Geometry check sheet. Reference: the model listing, model coordinates, mm. A direction names the side the tool comes from. Round coordinates to 2 decimals unless told otherwise and drop trailing zeros. Order: outer loops, then holes, each group sorted by start corner. A loop starts at its lowest first (then second) coordinate and runs counter-clockwise, first axis right, second up. Notation, with made-up numbers: (23, 66.5) -> (31, 66.5) arc R16 ccw to (31, 83.5) -> close; hole circle Ø4 at (85.5, -6). An arc over 180 degrees is marked (long way). Answer as a JSON object with one key per item and string values. Group by question number.
from build123d import *

# Parameters (mm, degrees)
SKETCH1_W                  = 127.078191072
SKETCH1_H                  = 113.282646321
BOSS_EXTRUDE1_DEPTH        = 39.624
SHELL_1_T                  = -2.54
OFFICIAL_RIB_BLOCK20_DEPTH = 2.54


# Read off the part's stored shape, not the designer's step: official_rib_block20
with BuildPart() as part:
    # Sketch1 → Boss-Extrude1 (new body)
    with BuildSketch(Plane(origin=(0, 0, 0), x_dir=(1, 0, 0), z_dir=(0, 1, 0))):
        with Locations((1.06119575, 7.295720781)):
            Rectangle(SKETCH1_W, SKETCH1_H)
    extrude(amount=BOSS_EXTRUDE1_DEPTH)

    # 抽壳1
    shell_1_openings = [part.faces().sort_by_distance(p)[0] for p in [
        (1.06119575, 39.624, -7.295720782),
    ]]
    offset(amount=SHELL_1_T, openings=shell_1_openings, kind=Kind.INTERSECTION)

    # official_rib_block20 outline → official_rib_block20 (add)
    with BuildSketch(Plane(origin=(0.729572078, 0, -0.729572078), x_dir=(0.7071067811865477, 0, 0.7071067811865475), z_dir=(-0.7071067811865475, 0, 0.7071067811865477))):
        Polygon((67.224888407, 33.535890054), (7.726, 25.357), (-34.23, 35.134), (-85.796761505, 21.08206499), (-86, 21.02668253), (-86, 2), (68, 2), (68, 33.642439145), align=None)
    extrude(amount=OFFICIAL_RIB_BLOCK20_DEPTH)


solid = part.part
Item 1: Sectioned sample at C-C, the plane x = 20. Enter the section's corners in (y, z), then the cut area to 3 significant figures.
Item 2: Set-up check for faces 5 (the flat face through (-9.319, 30.177, -9.007)), 6 (the flat face through (0, 20, 49.346)): record each of +Z, -Z, +X, -X, +Y, -Y from which the full face is reachable in a straight line by a thin tool's end or side.
Item 3: Sectioned sample at A-A, the plane y = 7. Enter the section's corners in (x, z).
Item 4: Thickness scan on L1, parallel to Z at x = 33, y = 14.5; L2, parallel to Z at x = 21.5, y = 8; L3, parallel to X at y = 9.5, z = 20. Record the ranges inside material, lowest first.
Item 5: Sectioned sample at D-D, the plane z = 22. Enter the section's corners in (x, y), then the cut area to 3 significant figures.
Item 6: Depth check by flat-ended pin: pin 1 Ø2 at (x, z) = (48.5, 26) entering from +Y. Enter the tip coordinate at first touch or a pass-through.
Item 7: Sectioned sample at B-B, the plane y = 27. Enter the section's corners in (x, z), then the cut area to 3 significant figures.
Item 8: Mould release check, pull along X, two halves, no side actions. Record for faces 1 (the flat face through (-59.938, 21, -7)), 2 (the flat face through (0, 20, -63.937)), 3 (the flat face through (-32, 2.54, 17)), 4 (the flat face through (64.6, 20, -7)): pulls with the +X half, pulls with the -X half, needs draft (parallel to the pull), parting line crosses it, or undercut.
Result:
{
 "1": {"outline": "(0, -63.94) -> (39.62, -63.94) -> (39.62, -61.4) -> (2.54, -61.4) -> (2.54, 18.54) -> (28.04, 18.54) -> (28.39, 22.13) -> (2.54, 22.13) -> (2.54, 46.81) -> (39.62, 46.81) -> (39.62, 49.35) -> (0, 49.35) -> close", "area": "568 mm2"},
 "2": {"face 5": "+Y", "face 6": "+Z, +X, -X, +Y, -Y"},
 "3": {"outline": "(-62.48, -63.94) -> (64.6, -63.94) -> (64.6, 49.35) -> (-62.48, 49.35) -> close; hole (-59.94, -61.4) -> (62.06, -61.4) -> (62.06, 46.81) -> (48.26, 46.81) -> close; hole (-59.94, -57.8) -> (44.67, 46.81) -> (-59.94, 46.81) -> close"},
 "4": {"L1": "z = -63.94 to -61.4, 31.54 to 35.13, 46.81 to 49.35", "L2": "z = -63.94 to -61.4, 20.04 to 23.63, 46.81 to 49.35", "L3": "x = -62.48 to -59.94, 17.87 to 21.46, 62.06 to 64.6"},
 "5": {"outline": "(-62.48, 0) -> (64.6, 0) -> (64.6, 39.62) -> (62.06, 39.62) -> (62.06, 2.54) -> (23.46, 2.54) -> (23.46, 28.71) -> (19.87, 28.36) -> (19.87, 2.54) -> (-59.94, 2.54) -> (-59.94, 39.62) -> (-62.48, 39.62) -> close", "area": "605 mm2"},
 "6": {"pin 1": "stops at y = 2.54"},
 "7": {"outline": "(-62.48, -63.94) -> (64.6, -63.94) -> (64.6, 49.35) -> (-62.48, 49.35) -> close; (-46.38, -44.24) -> (-44.58, -46.04) -> (1.21, -0.25) -> (-0.59, 1.54) -> close; hole (-59.94, -61.4) -> (62.06, -61.4) -> (62.06, 46.81) -> (48.26, 46.81) -> (14.64, 13.19) -> (12.85, 14.98) -> (44.67, 46.81) -> (-59.94, 46.81) -> close", "area": "1,480 mm2"},
 "8": {"face 1": "undercut", "face 2": "needs draft", "face 3": "undercut", "face 4": "pulls with the +X half"}
}
